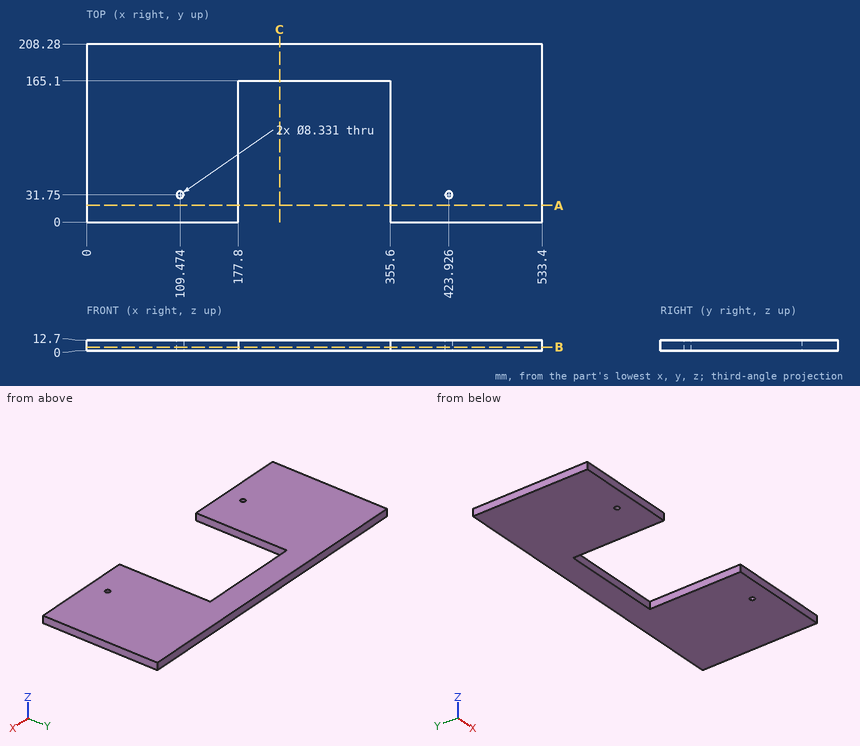
Study the drawing (mm; zero at the part's minimum x, y, z) and answer. Coordinates: 2 decimals unless noted, no trailing zeros. Write each loop counter-clockwise with the first axis right and the second up, starting at its lowest first coordinate (ties: lowest second). Pieces come first, ordered by that corner, then holes. Notation, with made-up numbers: M 75.5,4.5 L 125.5,4.5 A14 ccw 125.5,27.5 Z; hole C 41.5,-17 d10. An arc over 180 degrees is marked long. Use one line per item in the form item = value.
Item 1: Find the intervals of material crossed by probe 1 along X at (y, z) = (75, 12); probe 2 along Y at (x, z) = (337.5, 6); probe 3 along Y at (x, z) = (425, 3) (1 decimal), in increasing order.
Model answer:
probe_1 = 0 to 177.8, 355.6 to 533.4
probe_2 = 165.1 to 208.28
probe_3 = 0 to 27.7, 35.8 to 208.3
Item 2: Find section C-C, the plane x = 226. Give the vertices of the cut face in (y, z).
Model answer:
outline = M 165.1,0 L 208.28,0 L 208.28,12.7 L 165.1,12.7 Z
Item 3: Find section A-A, the plane y = 19.5. Give the vertices of the cut face in (x, z).
Model answer:
outline = M 0,0 L 177.8,0 L 177.8,12.7 L 0,12.7 Z; M 355.6,0 L 533.4,0 L 533.4,12.7 L 355.6,12.7 Z
Item 4: Find section B-B, the plane z = 4.5. Give the vertices of the cut face in (x, y).
Model answer:
outline = M 0,0 L 177.8,0 L 177.8,165.1 L 355.6,165.1 L 355.6,0 L 533.4,0 L 533.4,208.28 L 0,208.28 Z; hole C 109.47,31.75 d8.33; hole C 423.93,31.75 d8.33
Item 5: Given P1, Ø1, axis at x = 329, z = 7, coming from the -Y side; P2, Ø5, axis at x = 423.926, y = 31.75, coming from the -Z side, each flat-ended and moving along its own axis, determine where each tip first touches the part or whether it passes through.
Model answer:
P1 = 165.1
P2 = through
